CAD build for the part. Positions are in the model's coordinates, mm. Face numbers are marked on the shaded views. A direction names the side the tool comes from. Coordinates: 2 decimals unless noted, no trailing zeros. Loops run counter-clockwise (first coordinate to the right, second up) from the corner with the lowest first, then second, coordinate; pieces in that order, holes last. Notation, with made-up numbers: (-9, -19) -> (17, -19) arc R13 ccw to (17, -15) -> close; hole circle Ø8 at (45.25, -8). An arc over 180 degrees is marked (long way). Answer as CSV lines item,"result". Start each with the question number.
```python
from build123d import *

# Parameters (mm, degrees)
EXTRUDE_2_DEPTH     = 19
SKETCH_2_R          = 2.5
CUT_EXTRUDE_1_DEPTH = 107.646894001
SKETCH_3_R          = 2.5
CUT_EXTRUDE_2_DEPTH = 107.646894001


with BuildPart() as part:
    # 草图1 → 凸台-拉伸2 (new body)
    with BuildSketch(Plane(origin=(0, 0, 0), x_dir=(1, 0, 0), z_dir=(0, 1, 0))):
        with BuildLine():
            Line((75, 0), (8, 0))
            Line((8, 0), (0, -8))
            Line((0, -8), (0, -75))
            Line((0, -75), (1.6, -75))
            Line((1.6, -75), (1.6, -21.6))
            ThreePointArc((1.6, -21.6), (7.457864376, -7.457864376), (21.6, -1.6))
            Line((21.6, -1.6), (75, -1.6))
            Line((75, -1.6), (75, 0))
        make_face()
    extrude(amount=EXTRUDE_2_DEPTH)

    # 草图2 → 切除-拉伸1 (cut, through all)
    with BuildSketch(Plane.XY.offset(1.6)):
        with Locations((25, 9.5)):
            Circle(SKETCH_2_R)
        with Locations((65, 9.5)):
            Circle(SKETCH_2_R)
    extrude(amount=-CUT_EXTRUDE_1_DEPTH, mode=Mode.SUBTRACT)

    # 草图3 → 切除-拉伸2 (cut, through all)
    with BuildSketch(Plane(origin=(1.6, 0, 0), x_dir=(0, 0, -1), z_dir=(1, 0, 0))):
        with Locations((-65, 9.5)):
            Circle(SKETCH_3_R)
        with Locations((-25, 9.5)):
            Circle(SKETCH_3_R)
    extrude(amount=-CUT_EXTRUDE_2_DEPTH, mode=Mode.SUBTRACT)


solid = part.part
```
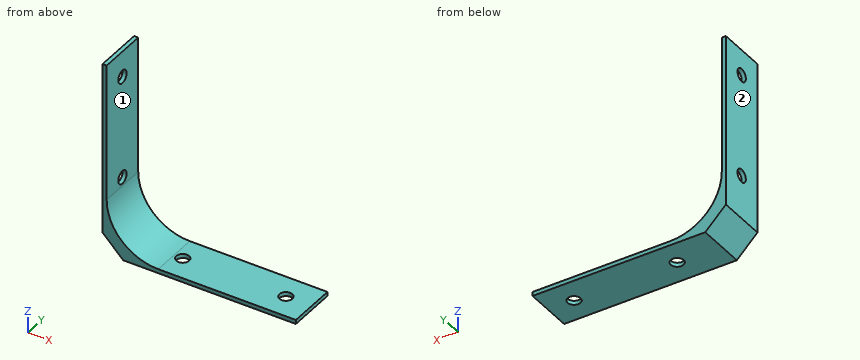
Q1. Saw through at B-B (z = 65). List the corners of the cut face in (x, y), and give its area (3 significant figures).
Q2. Which spindle directions (+Z, -Z, +X, -X, +Y, -Y) get a long thin tool onto all of the face, cutting with end or side? Do the marked faces 1 and 2. Say none if no direction does.
Q3. Pin check, flat tips, straight feed: pin 1 Ø2 at (y, z) = (9.5, 20) entering from +X; pin 2 Ø1.5 at (x, y) = (67, 8.5) entering from +Z; pin 3 Ø6 at (x, y) = (65, 9.5) entering from -Z; pin 4 Ø4 at (y, z) = (9.5, 25) entering from +X. Stop position of each tip, or through.
Q4. Saw through at A-A (x = 65). List the corners of the cut face in (y, z), and give its area (3 significant figures).
Q5. Saw through at C-C (y = 8). List the corners of the cut face in (x, z).
Q6. Probe probe 1 along Y at (x, z) = (1.05, 25); probe 2 along X at (y, z) = (6, 44). List the from-to ranges inside material, lowest first. Write a range as from..to.
Q7. Saw through at D-D (x = 53). List the corners of the cut face in (y, z), and give its area (3 significant figures).
Ans:
1,outline,"(0, 0) -> (1.6, 0) -> (1.6, 7) -> (0, 7) -> close; (0, 12) -> (1.6, 12) -> (1.6, 19) -> (0, 19) -> close"
1,area,"22.4 mm²"
2,face 1,"+Z, +X, +Y, -Y"
2,face 2,"+Z, -Z, -X, +Y, -Y"
3,pin 1,"stops at x = 1.77"
3,pin 2,"stops at z = 1.6"
3,pin 3,"stops at z = 0"
3,pin 4,"passes through"
4,outline,"(0, 0) -> (7, 0) -> (7, 1.6) -> (0, 1.6) -> close; (12, 0) -> (19, 0) -> (19, 1.6) -> (12, 1.6) -> close"
4,area,"22.4 mm²"
5,outline,"(0, 8) -> (8, 0) -> (23, 0) -> (23, 1.6) -> (21.6, 1.6) arc R20 cw to (1.6, 21.6) -> (1.6, 23) -> (0, 23) -> close; (0, 27) -> (1.6, 27) -> (1.6, 63) -> (0, 63) -> close; (0, 67) -> (1.6, 67) -> (1.6, 75) -> (0, 75) -> close; (27, 0) -> (63, 0) -> (63, 1.6) -> (27, 1.6) -> close; (67, 0) -> (75, 0) -> (75, 1.6) -> (67, 1.6) -> close"
6,probe 1,"y = 0..7, 12..19"
6,probe 2,"x = 0..1.6"
7,outline,"(0, 0) -> (19, 0) -> (19, 1.6) -> (0, 1.6) -> close"
7,area,"30.4 mm²"
